The model under review builds one solid part; all positions refer to its coordinate system, in mm. A direction names the side the tool comes from. Coordinates: 2 decimals unless noted, no trailing zeros. Order: outer loops, then holes, each group sorted by start corner. A loop starts at its lowest first (then second) coordinate and runs counter-clockwise, first axis right, second up. Notation, with made-up numbers: (-30.5, 44) - (16.5, 44) arc R14 ccw to (16.5, 59) - close; hole circle Ø2 at (-33.5, -21). An arc over 180 degrees is marked (long way). Answer in a Markdown table with one row per item.
```python
from build123d import *

# Parameters (mm, degrees)
F0_W     = 25.4
F0_H     = 25.4
F0_H_2   = 25.282406
F1_DEPTH = 25.4


with BuildPart() as f1:
    # F0 (on Front) → F1 (new body)
    with BuildSketch(Plane.XZ):
        with Locations((-38.1, 38.1)):
            Rectangle(F0_W, F0_H)
        with Locations((-38.1, 12.7)):
            Rectangle(F0_W, F0_H)
        with Locations((-38.1, -12.641203)):
            Rectangle(F0_W, F0_H_2)
        with Locations((-12.7, -12.641203)):
            Rectangle(F0_W, F0_H_2)
        Polygon((25.4, 0), (0, 0), (0, -25.282406), (0, -25.4), (25.4, -25.4), align=None)
        with Locations((12.7, 12.7)):
            Rectangle(F0_W, F0_H)
    extrude(amount=F1_DEPTH)


solid = f1.part
```
Item 1: We need section A-A, the plane z = 15.5. Write out the cut boundary in (x, y), then the cut area to 3 significant figures.
Check values:
| item | result |
|---|---|
| outline | (-50.8, -25.4) - (-25.4, -25.4) - (-25.4, 0) - (-50.8, 0) - close; (0, -25.4) - (25.4, -25.4) - (25.4, 0) - (0, 0) - close |
| area | 1,290 mm^2 |
Item 2: Mouldability with a two-part tool opening along X and no side actions: class faces 4 (the face through (0, -13, 13)), 5 (the face through (13, -13, 25.4)), 6 (the face through (-50.8, -13, 13)), 7 (the face through (-25.4, -13, 25)) as +X half, -X half, draft (parallel to the pull), parting line (faces both ways), or undercut.
Check values:
| item | result |
|---|---|
| face 4 | undercut |
| face 5 | draft |
| face 6 | -X half |
| face 7 | undercut |
Item 3: We need section B-B, the plane y = -17.75. Write out the cut boundary in (x, z), then the cut area to 3 significant figures.
Check values:
| item | result |
|---|---|
| outline | (-50.8, -25.28) - (0, -25.28) - (0, -25.4) - (25.4, -25.4) - (25.4, 25.4) - (0, 25.4) - (0, 0) - (-25.4, 0) - (-25.4, 50.8) - (-50.8, 50.8) - close |
| area | 3,860 mm^2 |
Item 4: We need section D-D, the plane z = 44.5. Write out the cut boundary in (x, y), then the cut area to 3 significant figures.
Check values:
| item | result |
|---|---|
| outline | (-50.8, -25.4) - (-25.4, -25.4) - (-25.4, 0) - (-50.8, 0) - close |
| area | 645 mm^2 |
Item 5: We need section C-C, the plane x = -15. Write out the cut boundary in (y, z), then the cut area to 3 significant figures.
Check values:
| item | result |
|---|---|
| outline | (-25.4, -25.28) - (0, -25.28) - (0, 0) - (-25.4, 0) - close |
| area | 642 mm^2 |
Item 6: Tool access review of faces 1 (the face through (-13, -13, 0)), 2 (the face through (-26, -13, -25.282)), 3 (the face through (-38, -13, 50.8)): name each direction out of +Z, -Z, +X, -X, +Y, -Y from which nothing blocks a thin tool from reaching the whole face with its end or side.
Check values:
| item | result |
|---|---|
| face 1 | +Z, +Y, -Y |
| face 2 | -Z, -X, +Y, -Y |
| face 3 | +Z, +X, -X, +Y, -Y |
Item 7: Clearance check with flat-ended pins moving along their axes: pin 1 Ø12.5 at (x, y) = (11.5, -13) entering from +Z; pin 2 Ø4 at (x, y) = (-23, -3.5) entering from +Z; pin 3 Ø12.5 at (x, y) = (-29, -10.5) entering from -Z. State where each tip first meets the part, or that it passes through.
Check values:
| item | result |
|---|---|
| pin 1 | z = 25.4 |
| pin 2 | z = 0 |
| pin 3 | z = -25.28 |
Item 8: To check wall thickness, follow line 1 (X direction, y = -11.5, z = 12.5); line 2 (X direction, y = -10.25, z = 28); line 3 (Z direction, x = -44, y = -19.5). State the ranges of each line that lie inside material, in increasing order. Write a range as from..to.
Check values:
| item | result |
|---|---|
| line 1 | -50.8..-25.4, 0..25.4 |
| line 2 | -50.8..-25.4 |
| line 3 | -25.28..50.8 |
